The drawing under review shows one solid part. Ordinate dimensions are in mm from its lowest x, y, z. Round coordinates to 2 decimals unless told otherwise and drop trailing zeros. Order: outer loops, then holes, each group sorted by start corner. A loop starts at its lowest first (then second) coordinate and runs counter-clockwise, first axis right, second up. Notation, with made-up numbers: (-39.5, 66.25) -> (3.5, 66.25) arc R10 cw to (3.5, 80.25) -> close; hole circle Ø11 at (25.25, 44.5). An arc over 180 degrees is marked (long way). Use a Markdown table: item, result. Add a question column.
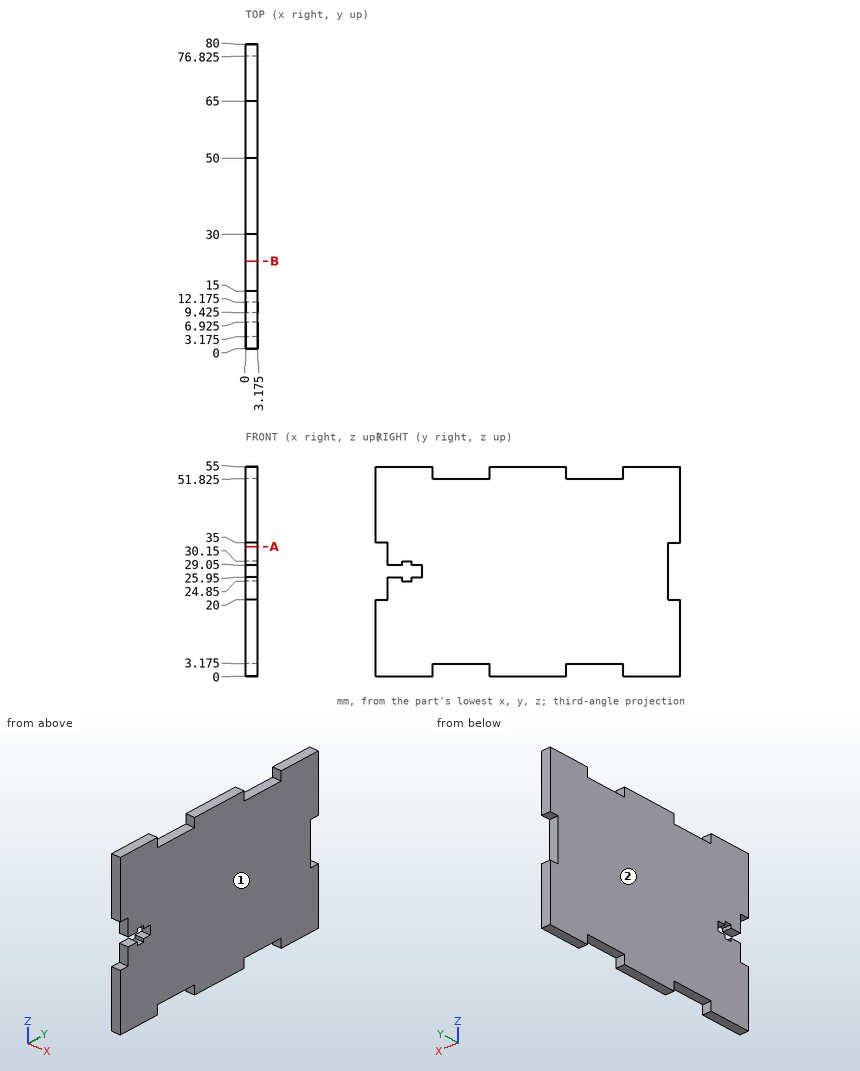
Q1. Add section A-A, the plane z = 34. Give the boundary of the cut face in (x, y) (3 decimals).
Q2. To check wall thickness, follow line 1 along Y through (x, z) = (2.95, 52); line 2 along Z through (x, y) = (0.8, 9.5); line 3 along Y through (x, z) = (2.55, 20.5) (3 decimals). State the ranges of each line that lie inside material, in increasing order.
Q3. Add section B-B, the plane y = 23. Give the boundary of the cut face in (x, z) (3 decimals), then the cut area to 3 significant figures.
Q4. Draft analysis for pull direction X (two halves, no side actions). For the marked faces 1 and 2, state which applies: released by +X, released by -X, zero draft, split by the parting line, or undercut.
Q5. For pin 1 (1.6 mm diameter, centred on x = 1, z = 27.5, fed in from +Y) (3 decimals); pin 2 (0.9 mm diameter, centred on x = 1, z = 28, fed in from -Y) (3 decimals), all flat-tipped, find the tip position at first contact; note any pin that passes through.
Return value:
| question | item | result |
|---|---|---|
| 1 | outline | (0, 3.175) -> (3.175, 3.175) -> (3.175, 76.825) -> (0, 76.825) -> close |
| 2 | line 1 | 0 to 15, 30 to 50, 65 to 80 |
| 2 | line 2 | 0 to 25.95, 29.05 to 55 |
| 2 | line 3 | 3.175 to 76.825 |
| 3 | outline | (0, 3.175) -> (3.175, 3.175) -> (3.175, 51.825) -> (0, 51.825) -> close |
| 3 | area | 154 mm² |
| 4 | face 1 | released by +X |
| 4 | face 2 | released by -X |
| 5 | pin 1 | y = 76.825 |
| 5 | pin 2 | y = 12.175 |
